Input: part model. Units: mm. Frame: model coordinates. A direction names the side the tool comes from. Give positions to 0.01 mm unless a question says otherwise; leave off trailing zeros. Order: outer loops, then holes, each group sorted by start corner. A loop starts at its lowest first (then second) coordinate and runs counter-clockwise, first axis right, second up. Notation, with made-up numbers: (-22.5, 71.25) - (-2.5, 71.25) arc R8 ccw to (-2.5, 77.25) - close; hole circle Ø2 at (-4.75, 38.25). An arc over 180 degrees is marked (long way). Use a Markdown table: item, result.
from build123d import *

# Parameters (mm, degrees)
SKETCH_1_W              = 53
SKETCH_1_H              = 50
EXTRUDE_1_DEPTH         = 3
CHAMFER_1_SIZE          = 5
CUT_EXTRUDE_1_REACH     = 38.555
SKETCH_3_W              = 3
SKETCH_3_H              = 50
EXTRUDE_2_DEPTH         = 51
FILLET_1_R              = 2
RIB_1_REACH             = 80.219
SKETCH_6_WALL_W         = 182.292207198
SKETCH_6_WALL_H         = 3
RIB_3_REACH             = 80.219
SKETCH_8_WALL_W         = 182.292207198
SKETCH_8_WALL_H         = 3
CHAMFER_2_SIZE          = 5
CUT_EXTRUDE_2_REACH     = 79.724
SKETCH_9_R              = 11.05
HOLE_WIZARD_3_5_3_5_1_D = 3.5


with BuildPart() as part:
    # 草图1 → 凸台-拉伸1 (new body)
    with BuildSketch(Plane(origin=(0, 0, 0), x_dir=(1, 0, 0), z_dir=(0, 1, 0))):
        Rectangle(SKETCH_1_W, SKETCH_1_H)
    extrude(amount=EXTRUDE_1_DEPTH)

    # 倒角1
    chamfer_1_edges = [part.edges().sort_by_distance(p)[0] for p in [
        (26.5, 1.5, 25),
        (26.5, 1.5, -25),
    ]]
    chamfer(chamfer_1_edges, length=CHAMFER_1_SIZE)

    # 草图2 → 切除-拉伸1 (cut, up to next)
    with BuildSketch(Plane(origin=(0, 3, 0), x_dir=(1, 0, 0), z_dir=(0, 1, 0)), mode=Mode.PRIVATE) as cut_extrude_1_sk1:
        with BuildLine():
            Line((-14.5, 17.1), (15.5, 17.1))
            ThreePointArc((15.5, 17.1), (17.6, 15), (15.5, 12.9))
            Line((15.5, 12.9), (-14.5, 12.9))
            ThreePointArc((-14.5, 12.9), (-16.6, 15), (-14.5, 17.1))
        make_face()
    cut_extrude_1_tool1 = extrude(cut_extrude_1_sk1.sketch, amount=-CUT_EXTRUDE_1_REACH, mode=Mode.PRIVATE) & part.part
    # 草图2 → 切除-拉伸1 (cut, up to next)
    with BuildSketch(Plane(origin=(0, 3, 0), x_dir=(1, 0, 0), z_dir=(0, 1, 0)), mode=Mode.PRIVATE) as cut_extrude_1_sk2:
        with BuildLine():
            Line((-14.5, -12.9), (15.5, -12.9))
            ThreePointArc((15.5, -12.9), (17.6, -15), (15.5, -17.1))
            Line((15.5, -17.1), (-14.5, -17.1))
            ThreePointArc((-14.5, -17.1), (-16.6, -15), (-14.5, -12.9))
        make_face()
    cut_extrude_1_tool2 = extrude(cut_extrude_1_sk2.sketch, amount=-CUT_EXTRUDE_1_REACH, mode=Mode.PRIVATE) & part.part
    add(cut_extrude_1_tool1.solids().sort_by_distance((0.5, 3, -15))[0], mode=Mode.SUBTRACT)
    add(cut_extrude_1_tool2.solids().sort_by_distance((0.5, 3, 15))[0], mode=Mode.SUBTRACT)

    # 草图3 → 凸台-拉伸2 (add)
    with BuildSketch(Plane(origin=(0, 3, 0), x_dir=(1, 0, 0), z_dir=(0, 1, 0))):
        with Locations((-25, 0)):
            Rectangle(SKETCH_3_W, SKETCH_3_H)
    extrude(amount=EXTRUDE_2_DEPTH)

    # 圆角1
    fillet_1_edges = [part.edges().sort_by_distance(p)[0] for p in [
        (-26.5, 0, 0),
        (-23.5, 3, 0),
    ]]
    fillet(fillet_1_edges, radius=FILLET_1_R)

    # 草图6 wall → 筋1 (add, up to next)
    with BuildSketch(Plane(origin=(-17, 13, 25), x_dir=(0.544988350595, -0.838443616301, 0), z_dir=(0.838443616301, 0.544988350595, 0)), mode=Mode.PRIVATE) as rib_1_sk1:
        with Locations((0, 1.5)):
            Rectangle(SKETCH_6_WALL_W, SKETCH_6_WALL_H)
    rib_1_tool1 = extrude(rib_1_sk1.sketch, amount=-RIB_1_REACH, mode=Mode.PRIVATE) - part.part
    add(rib_1_tool1.solids().sort_by_distance((-17, 13, 25))[0])

    # 草图8 wall → 筋3 (add, up to next)
    with BuildSketch(Plane(origin=(-17, 13, -25), x_dir=(-0.544988350595, 0.838443616301, 0), z_dir=(0.838443616301, 0.544988350595, 0)), mode=Mode.PRIVATE) as rib_3_sk1:
        with Locations((0, 1.5)):
            Rectangle(SKETCH_8_WALL_W, SKETCH_8_WALL_H)
    rib_3_tool1 = extrude(rib_3_sk1.sketch, amount=-RIB_3_REACH, mode=Mode.PRIVATE) - part.part
    add(rib_3_tool1.solids().sort_by_distance((-17, 13, -25))[0])

    # 倒角2
    chamfer_2_edges = [part.edges().sort_by_distance(p)[0] for p in [
        (-25, 54, 25),
        (-25, 54, -25),
    ]]
    chamfer(chamfer_2_edges, length=CHAMFER_2_SIZE)

    # 草图9 → 切除-拉伸2 (cut, up to next)
    with BuildSketch(Plane(origin=(-23.5, 0, 0), x_dir=(0, 0, -1), z_dir=(1, 0, 0)), mode=Mode.PRIVATE) as cut_extrude_2_sk1:
        with Locations((0, 33)):
            Circle(SKETCH_9_R)
    cut_extrude_2_tool1 = extrude(cut_extrude_2_sk1.sketch, amount=-CUT_EXTRUDE_2_REACH, mode=Mode.PRIVATE) & part.part
    add(cut_extrude_2_tool1.solids().sort_by_distance((-23.5, 33, 0))[0], mode=Mode.SUBTRACT)

    # Ø3.5 (3.5) 直径孔1 (through all)
    with Locations(Plane(origin=(-23.5, 0, 0), x_dir=(0, 0, -1), z_dir=(1, 0, 0))):
        with Locations((-15.5, 48.5), (-15.5, 17.5), (15.5, 17.5), (15.5, 48.5)):
            Hole(HOLE_WIZARD_3_5_3_5_1_D / 2)


solid = part.part
1. Section query C-C (y = 24). Return loops of the section in (x, z), then the cut area to 3 significant figures.
Response:
| item | result |
|---|---|
| outline | (-26.5, -25) - (-23.5, -25) - (-23.5, -6.41) - (-26.5, -6.41) - close; (-26.5, 6.41) - (-23.5, 6.41) - (-23.5, 25) - (-26.5, 25) - close |
| area | 112 mm^2 |
2. Set-up query: faces 4 (the face through (1, 2, 17.1)), 5 (the face through (-17, 13, 23)), 6 (the face through (-19, 9, -22)). Return all of +Z, -Z, +X, -X, +Y, -Y with unobstructed straight access to the full face (end or side cutting, diameter ignored); none if empty.
Response:
| item | result |
|---|---|
| face 4 | +Y, -Y |
| face 5 | +Z, -Z, +X, +Y |
| face 6 | +X, +Y |
3. Mould query, pull axis Z, two halves, no side actions, for faces 1 (the face through (17.6, 1.5, 15)), 2 (the face through (24, 1.5, -22.5)), 3 (the face through (-25, 54, 0)). Classes: pulls with the +Z half, pulls with the -Z half, needs draft (parallel to the pull), parting line crosses it, or undercut.
Response:
| item | result |
|---|---|
| face 1 | undercut |
| face 2 | pulls with the -Z half |
| face 3 | needs draft |
4. Material intervals for line 1 along Y through (x, z) = (-24.55, -15.5); line 2 along Y through (x, z) = (-25.5, -15.5); line 3 along Z through (x, y) = (-24, 17), sorted ascending.
Response:
| item | result |
|---|---|
| line 1 | y = 0 to 15.75, 19.25 to 46.75, 50.25 to 54 |
| line 2 | y = 0.27 to 15.75, 19.25 to 46.75, 50.25 to 54 |
| line 3 | z = -25 to -17.18, -13.82 to 13.82, 17.18 to 25 |
5. Pin query (flat end, axial travel): pin 1 (4 mm diameter, centred on y = 17.5, z = 15.5, fed in from +X). Return the tip coordinate at first contact, or that it passes through.
Response:
| item | result |
|---|---|
| pin 1 | stops at x = -23.5 |
6. Section query A-A (z = 0). Return loops of the section in (x, y), then the cut area to 3 significant figures.
Response:
| item | result |
|---|---|
| outline | (-26.5, 2) arc R2 ccw to (-24.5, 0) - (26.5, 0) - (26.5, 3) - (-21.5, 3) arc R2 cw to (-23.5, 5) - (-23.5, 21.95) - (-26.5, 21.95) - close; (-26.5, 44.05) - (-23.5, 44.05) - (-23.5, 54) - (-26.5, 54) - close |
| area | 246 mm^2 |
7. Section query B-B (x = 8.5). Return loops of the section in (y, z).
Response:
| item | result |
|---|---|
| outline | (0, -25) - (3, -25) - (3, -17.1) - (0, -17.1) - close; (0, -12.9) - (3, -12.9) - (3, 12.9) - (0, 12.9) - close; (0, 17.1) - (3, 17.1) - (3, 25) - (0, 25) - close |
8. Section query D-D (z = -18). Return loops of the section in (x, y).
Response:
| item | result |
|---|---|
| outline | (-26.5, 2) arc R2 ccw to (-24.5, 0) - (26.5, 0) - (26.5, 3) - (-21.5, 3) arc R2 cw to (-23.5, 5) - (-23.5, 54) - (-26.5, 54) - close |
